Answer from the drawing. Dimensions are ordinates in mm from the lowest x, y and z of the part. A direction names the side the tool comes from. Coordinates: 2 decimals unless noted, no trailing zeros. Loops run counter-clockwise (first coordinate to the right, second up) from the corner with the lowest first, then second, coordinate; pieces in that order, holes last. Notation, with made-up numbers: (76, -35) -> (97, -35) arc R16 cw to (97, -22) -> close; hole circle Ø6 at (22.5, 80). An arc over 180 degrees is marked (long way). Answer as CSV lines item,"result".
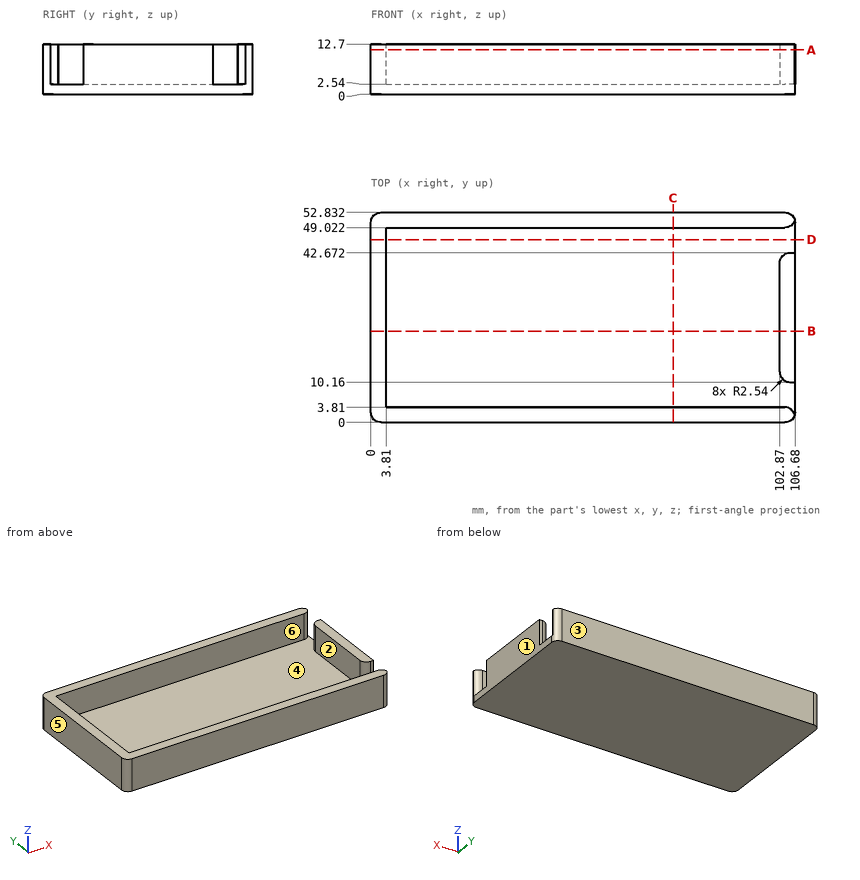
(1) A cutting plane is placed at D-D, the plane y = 46. Write down the section's boundary in (x, z), and give its area (3 significant figures).
Computed values:
outline,"(0, 0) -> (106.68, 0) -> (106.68, 2.54) -> (3.81, 2.54) -> (3.81, 12.7) -> (0, 12.7) -> close"
area,"310 mm2"
(2) Which of the six approach directions +Z, -Z, +X, -X, +Y, -Y give full straight-line access (tool end or side, diameter ignored) to the marked faces 1 and 2?
Computed values:
face 1,"+Z, -Z, +X, +Y, -Y"
face 2,"+Z"
(3) A cutting plane is placed at C-C, the plane x = 76. Write down the section's boundary in (y, z), and give its area (3 significant figures).
Computed values:
outline,"(0, 0) -> (52.83, 0) -> (52.83, 12.7) -> (49.02, 12.7) -> (49.02, 2.54) -> (3.81, 2.54) -> (3.81, 12.7) -> (0, 12.7) -> close"
area,"212 mm2"
(4) Flat-ended cylindrical pins translate along their axes: pin 1 Ø24.5 at (x, y) = (72, 21.5) entering from +Z; pin 2 Ø1 at (x, z) = (106, 6) entering from +Y. Find the tip coordinate at first contact, or state that the pin passes through.
Computed values:
pin 1,"z = 2.54"
pin 2,"y = 52.44"
(5) A cutting plane is placed at B-B, the plane y = 23. Write down the section's boundary in (x, z), and give its area (3 significant figures).
Computed values:
outline,"(0, 0) -> (106.68, 0) -> (106.68, 12.7) -> (102.87, 12.7) -> (102.87, 2.54) -> (3.81, 2.54) -> (3.81, 12.7) -> (0, 12.7) -> close"
area,"348 mm2"
(6) For a pull along Y with two mould halves and no side action, classify the marked faces 3, 4, 5 and 6 as pulls with the +Y half, pulls with the -Y half, needs draft (parallel to the pull), parting line crosses it, or undercut.
Computed values:
face 3,"pulls with the +Y half"
face 4,"undercut"
face 5,"needs draft"
face 6,"undercut"
(7) A cutting plane is placed at A-A, the plane z = 11.25. Write down the section's boundary in (x, y) (3 decimals).
Computed values:
outline,"(0, 2.54) arc R2.54 ccw to (2.54, 0) -> (104.14, 0) arc R2.54 ccw to (106.599, 1.905) arc R2.54 ccw to (104.14, 3.81) -> (3.81, 3.81) -> (3.81, 49.022) -> (104.14, 49.022) arc R2.54 ccw to (106.599, 50.927) arc R2.54 ccw to (104.14, 52.832) -> (2.54, 52.832) arc R2.54 ccw to (0, 50.292) -> close; (102.87, 12.7) arc R2.54 ccw to (105.41, 10.16) -> (106.68, 10.16) -> (106.68, 42.672) -> (105.41, 42.672) arc R2.54 ccw to (102.87, 40.132) -> close"
(8) Consider line 1 along X through (y, z) = (19, 4); line 2 along Y through (x, z) = (66, 8.75); line 3 along Z through (x, y) = (80.5, 48). Determine where each line is inside the solid, lowest interval first.
Computed values:
line 1,"0 to 3.81, 102.87 to 106.68"
line 2,"0 to 3.81, 49.02 to 52.83"
line 3,"0 to 2.54"
